Geometry check sheet. Reference: the model listing, model coordinates, mm. A direction names the side the tool comes from. Give positions to 0.01 mm unless a question says otherwise; leave off trailing zeros. Write each loop counter-clockwise with the first axis right and the second up, starting at its lowest first coordinate (ties: lowest second). Pieces come first, ordered by that corner, then holes. Notation, with made-up numbers: (-29, 0) -> (-11, 0) arc R15 ccw to (-11, 25) -> close; hole circle Ø8 at (67, 87). An arc over 180 degrees is marked (long way). Write item = value, one per line. Start each with the question number.
1. Cross-section at D-D, the plane y = -4.5. Record the cut outline in (x, z), plus the area to 3 significant figures.
2. Set-up check for faces 1 (the flat face through (17.4, 7, 0)), 2 (the flat face through (-3.31, 2.24, 2.37)), 3 (the flat face through (-19, 6, 0)), 4 (the flat face through (19, 7, 2.85)): record each of +Z, -Z, +X, -X, +Y, -Y from which the full face is reachable in a straight line by a thin tool's end or side.
3. Thickness scan on line 1 along Z through (x, y) = (-1, -5.5); line 2 along Z through (x, y) = (1, -1.25); line 3 along Y through (x, z) = (-18, -7.75). Record the ranges inside material, lowest first.
4. Cross-section at A-A, the plane y = 3.75. Record the cut outline in (x, z), plus the area to 3 significant figures.
5. Cross-section at C-C, the plane z = -0.5. Record the cut outline in (x, y).
6. Depth check by flat-ended pin: P1, Ø6.5, axis at y = 7.5, z = 0.5, coming from the +X side; P2, Ø2, axis at y = -2, z = 8, coming from the +X side; P3, Ø3, axis at x = 20, y = 3.5, coming from the +Z side; P4, Ø3.5, axis at x = 2.5, y = -7, coming from the +Z side. Enter the tip coordinate at first touch or a pass-through.
7. Cross-section at B-B, the plane x = -16. Record the cut outline in (y, z).
8. Mould release check, pull along X, two halves, no side actions. Record for faces 5 (the flat face through (21, 4.5, 0)), 6 (the flat face through (-23.15, 4, 0)), 7 (the flat face through (-22, 1.6, 0)): pulls with the +X half, pulls with the -X half, needs draft (parallel to the pull), parting line crosses it, or undercut.
Autodesk Inventor part; units mm, degrees
ref_plane "Work Plane1" through (21.45, 1.6, 0) normal (0, 0, -1) x (-1, 0, 0)
ref_plane "YZ Plane" through (0, 0, 0) normal (1, 0, 0) x (0, 1, 0)
ref_plane "XZ Plane" through (0, 0, 0) normal (0, 1, 0) x (-1, 0, 0)
sketch "Sketch1" plane through (0, 0, 0) normal (0, 1, 0) x (-1, 0, 0)
  line L0 (-21.45, 8.75) -> (21.45, 8.75)
  line L1 (21.45, 8.75) -> (21.45, -8.75)
  line L2 (21.45, -8.75) -> (-21.45, -8.75)
  line L3 (-21.45, -8.75) -> (-21.45, 8.75)
  line L4 (-21.45, 8.75) -> (21.45, -8.75) construction
  line L5 (21.45, 8.75) -> (-21.45, -8.75) construction
  point P0 (0, 0)
  dimension "d0" = 42.9
  dimension "d1" = 17.5
extrude "Extrusion1" add sketch "Sketch1" along normal blind 1.6
sketch "Sketch2" plane through (0, 0, 0) normal (0, -1, 0) x (1, 0, 0)
  line L0 (21.45, -8.75) -> (-21.45, -8.75)
  line L1 (-21.45, -8.75) -> (-19.05, -8.75)
  line L2 (-19.05, -8.75) -> (18.75, -8.75)
  line L3 (18.75, -8.75) -> (18.75, -6.25)
  line L4 (18.75, -6.25) -> (-19.05, -6.25)
  line L5 (-19.05, -6.25) -> (-19.05, -8.75)
  point P0 (0, 0)
  dimension "d4" = 2.4
  dimension "d5" = 37.8
  dimension "d6" = 2.5
extrude "Extrusion2" add sketch "Sketch2" along normal blind 3
ref_plane "Work Plane1" through (21.45, 1.6, 0) normal (0, 0, -1) x (-1, 0, 0)
sketch "Sketch3" plane through (0, -3, 0) normal (0, -1, 0) x (1, 0, 0)
  line L0 (18.75, -6.25) -> (-19.05, -6.25)
  line L1 (-19.05, -8.75) -> (18.75, -8.75)
  line L2 (18.75, -6.25) -> (-19.05, -8.75)
  line L3 (18.75, -8.75) -> (-19.05, -6.25)
  line L4 (-18.2, -7.2) -> (17.9, -7.2)
  line L5 (17.9, -7.2) -> (17.9, -7.8)
  line L6 (17.9, -7.8) -> (-18.2, -7.8)
  line L7 (-18.2, -7.8) -> (-18.2, -7.2)
  line L8 (-18.2, -7.2) -> (17.9, -7.8) construction
  line L9 (17.9, -7.2) -> (-18.2, -7.8) construction
  point P0 (0, 0)
  point P1 (-0.15, -7.5)
  dimension "d10" = 36.1
  dimension "d11" = 0.6
extrude "Extrusion3" add sketch "Sketch3" along normal blind 6.8 contours L4 L5 L6 L3 L2 | L2 L3 L4 | L3 L2 L6 L7 L4 | L3 L6 L2
mirror "Mirror1" about plane through (21.45, 1.6, 0) normal (0, 0, -1) of "Extrusion3", "Extrusion2"
sketch "Sketch4" plane through (0, 1.6, 0) normal (0, 1, 0) x (1, 0, 0)
  line L0 (-21.45, 8.75) -> (-21.45, -8.75)
  line L1 (-10.5583, 0) -> (-5.75, 4.8083)
  line L2 (-5.75, 4.8083) -> (-0.9417, 0)
  line L3 (-0.9417, 0) -> (-5.75, -4.8083)
  line L4 (-5.75, -4.8083) -> (-10.5583, 0)
  point P0 (0, 0)
  point P1 (-5.75, 0)
  dimension "d15" = 6.8
extrude "Extrusion4" add sketch "Sketch4" along normal blind 1.3
sketch "Sketch5" plane through (0, 1.6, 0) normal (0, 1, 0) x (1, 0, 0)
  line L0 (21.45, -8.75) -> (21.45, 8.75)
  line L1 (21.45, -3.7) -> (16.45, -3.7)
  line L2 (16.45, -3.7) -> (16.45, 3.7)
  line L3 (16.45, 3.7) -> (21.45, 3.7)
  line L4 (21.45, 3.7) -> (21.45, -3.7)
  line L5 (21.45, -3.7) -> (16.45, 3.7) construction
  line L6 (16.45, -3.7) -> (21.45, 3.7) construction
  point P0 (0, 0)
  dimension "d19" = 5
  dimension "d20" = 7.4
extrude "Extrusion5" add sketch "Sketch5" along normal blind 2.9
sketch "Sketch6" plane through (0, 4.5, 0) normal (0, 1, 0) x (1, 0, 0)
  line L0 (16.45, -3.7) -> (21.45, -3.7)
  line L1 (21.45, -8.75) -> (21.45, 8.75)
  line L2 (21.45, 3.7) -> (16.45, 3.7)
  line L3 (20.5, -2.85) -> (17.4, -2.85)
  line L4 (17.4, -2.85) -> (17.4, 2.85)
  line L5 (17.4, 2.85) -> (20.5, 2.85)
  line L6 (20.5, 2.85) -> (20.5, -2.85)
  line L7 (20.5, -2.85) -> (17.4, 2.85) construction
  line L8 (17.4, -2.85) -> (20.5, 2.85) construction
  point P0 (0, 0)
  point P1 (18.95, 0)
  dimension "d23" = 3.1
  dimension "d24" = 5.7
extrude "Extrusion6" add sketch "Sketch6" along normal blind 5.7
sketch "Sketch7" plane through (0, 1.6, 0) normal (0, 1, 0) x (1, 0, 0)
  line L0 (-21.45, 8.75) -> (-21.45, -8.75)
  line L1 (-13.95, 4) -> (-23.15, 4)
  line L2 (-23.15, 4) -> (-23.15, -4)
  line L3 (-23.15, -4) -> (-13.95, -4)
  line L4 (-13.95, -4) -> (-13.95, 4)
  point P0 (0, 0)
  dimension "d29" = 9.2
  dimension "d30" = 8
extrude "Extrusion7" add sketch "Sketch7" along normal blind 4.4
properties part number "Arduino"
Answers:
q1.outline = (-18.2, -7.8) -> (17.9, -7.8) -> (17.9, -7.2) -> (-18.2, -7.2) -> close; (-18.2, 7.2) -> (17.9, 7.2) -> (17.9, 7.8) -> (-18.2, 7.8) -> close
q1.area = 43.3 mm^2
q2.face_1 = +Z, -Z, +Y
q2.face_2 = +Z, +Y
q2.face_3 = +Z, -Z, -X, +Y
q2.face_4 = +Z, +X, +Y
q3.line_1 = -7.8 to -7.2, 7.2 to 7.8
q3.line_2 = -8.75 to -6.25, 6.25 to 8.75
q3.line_3 = -9.8 to 1.6
q4.outline = (-23.15, -4) -> (-13.95, -4) -> (-13.95, 4) -> (-23.15, 4) -> close; (16.45, -3.7) -> (21.45, -3.7) -> (21.45, 3.7) -> (16.45, 3.7) -> close
q4.area = 111 mm^2
q5.outline = (-23.15, 1.6) -> (-21.45, 1.6) -> (-21.45, 0) -> (21.45, 0) -> (21.45, 4.5) -> (20.5, 4.5) -> (20.5, 10.2) -> (17.4, 10.2) -> (17.4, 4.5) -> (16.45, 4.5) -> (16.45, 1.6) -> (-1.44, 1.6) -> (-1.44, 2.9) -> (-10.06, 2.9) -> (-10.06, 1.6) -> (-13.95, 1.6) -> (-13.95, 6) -> (-23.15, 6) -> close
q6.P1 = 21.45
q6.P2 = 18.75
q6.P3 = 3.7
q6.P4 = 7.8
q7.outline = (-9.8, -7.8) -> (-3, -7.8) -> (-3, -8.75) -> (1.6, -8.75) -> (1.6, -4) -> (6, -4) -> (6, 4) -> (1.6, 4) -> (1.6, 8.75) -> (-3, 8.75) -> (-3, 7.8) -> (-9.8, 7.8) -> (-9.8, 7.2) -> (-3, 7.2) -> (-3, 6.25) -> (0, 6.25) -> (0, -6.25) -> (-3, -6.25) -> (-3, -7.2) -> (-9.8, -7.2) -> close
q8.face_5 = undercut
q8.face_6 = pulls with the -X half
q8.face_7 = needs draft
